Here's how the part is built. I have some questions about the finished solid (model axes, mm). Face numbers are marked on the shaded views. A direction names the side the tool comes from. Round coordinates to 2 decimals unless told otherwise and drop trailing zeros. Loops run counter-clockwise (first coordinate to the right, second up) from the corner with the lowest first, then second, coordinate; pieces in that order, holes last. Notation, with made-up numbers: (-2, 50.5) - (26, 50.5) arc R26 ccw to (26, 86.5) - close; hole circle Ø11 at (50, 57.5). An arc over 180 degrees is marked (long way). Return JSON: item names as keys, results as strings. Group by question number.
Autodesk Inventor part; units mm, degrees
ref_plane "YZ Plane" through (0, 0, 0) normal (1, 0, 0) x (0, 1, 0)
ref_plane "XZ Plane" through (0, 0, 0) normal (0, 1, 0) x (-1, 0, 0)
ref_plane "XY Plane" through (0, 0, 0) normal (0, 0, 1) x (1, 0, 0)
sketch "Sketch1" plane through (0, 0, 0) normal (0, 0, 1) x (1, 0, 0)
  line L0 (0, 0) -> (-61.1827, -8.0012) construction
  line L1 (61.2899, -8.1227) -> (0, 0) construction
  line L2 (86.7988, -11.5034) -> (67.2983, -8.919)
  line L3 (-67.1847, -8.7862) -> (-86.5468, -11.3183)
  line L4 (0, 0) -> (0, -62.0753) construction
  line L5 (61.2899, -8.1227) -> (0, -62.0753) construction
  line L6 (-61.1827, -8.0012) -> (0, -62.0753) construction
  arc A0 (-29.7125, -39.3071) -> (-39.2375, -29.7799) centre (-39.2375, -39.3049) ccw
  arc A1 (-60.1692, -13.6752) -> (-55.9036, -26.1177) centre (0, 0) ccw
  arc A2 (56.0545, -26.1271) -> (60.2727, -13.8035) centre (0.1394, -0.1047) ccw
  line L7 (-50.1505, -29.7799) -> (-39.2375, -29.7799)
  line L8 (-29.7125, -39.3071) -> (-29.7151, -50.2201)
  arc A3 (39.3667, -29.7672) -> (29.6251, -39.4816) centre (39.3395, -39.4816) ccw
  line L9 (29.6251, -39.4816) -> (29.6251, -50.3946)
  line L10 (39.3667, -29.7672) -> (50.2797, -29.7978)
  circle A4 centre (0.1394, -0.1047) radius 55.5625 construction
  line L11 (-39.2375, -39.3049) -> (0.1394, -0.1047) construction
  line L12 (0.1394, -0.1047) -> (39.3395, -39.4816) construction
  line L13 (39.3395, -39.4816) -> (0, -62.0753) construction
  line L14 (-39.2375, -39.3049) -> (0, -62.0753) construction
  circle A5 centre (-39.2375, -39.3049) radius 2.4384
  circle A6 centre (39.3395, -39.4816) radius 2.4384
  arc A7 (-91.9453, -18.8835) -> (-85.1324, -39.6138) centre (0.1394, -0.1047) ccw
  arc A8 (-76.9964, -53.7918) -> (-8.2199, -93.7122) centre (0.1394, -0.1047) ccw
  arc A9 (8.2102, -93.7375) -> (77.1094, -54.0293) centre (0.1394, -0.1047) ccw
  arc A10 (83.8051, -42.9099) -> (92.1837, -19.0805) centre (0.1394, -0.1047) ccw
  line L15 (-93.0629, -12.1704) -> (-83.6165, -42.7332) construction
  line L16 (-78.9151, -50.9242) -> (-4.7625, -93.9568) construction
  line L17 (4.7625, -93.9709) -> (79.0426, -51.1588) construction
  line L18 (83.8051, -42.9099) -> (93.316, -12.3671) construction
  line L19 (0, -62.0753) -> (0, -103.9027) construction
  line L20 (-4.7625, -90.5498) -> (-4.7625, -86.0193)
  line L21 (4.7625, -86.0193) -> (4.7625, -90.5743)
  arc A11 (4.7625, -86.0193) -> (-4.7625, -86.0193) centre (0, -86.0193) ccw
  line L22 (0.1394, -0.1047) -> (81.6013, -47.1368) construction
  line L23 (83.8051, -42.9099) -> (76.9144, -38.9315)
  line L24 (72.1519, -47.1804) -> (76.0966, -49.4579)
  arc A12 (76.9144, -38.9315) -> (72.1519, -47.1804) centre (74.5331, -43.0559) ccw
  line L25 (0.1394, -0.1047) -> (-92.6905, -53.7001) construction
  line L26 (-80.6641, -41.0286) -> (-76.7766, -38.7842)
  line L27 (-72.0545, -46.9632) -> (-75.978, -49.2284)
  arc A13 (-72.0545, -46.9632) -> (-76.7766, -38.7842) centre (-74.4155, -42.8737) ccw
  arc A14 (-86.5468, -11.3183) -> (-91.9453, -18.8835) centre (-85.7234, -17.6146) ccw
  arc A15 (-60.1692, -13.6752) -> (-67.1847, -8.7862) centre (-66.3613, -15.0825) ccw
  arc A16 (-55.9036, -26.1177) -> (-50.1505, -29.7799) centre (-50.1505, -23.4299) ccw
  arc A17 (-29.7151, -50.2201) -> (-25.945, -56.0239) centre (-23.3651, -50.2216) ccw
  arc A18 (25.7485, -56.2431) -> (29.6251, -50.3946) centre (23.2751, -50.3946) ccw
  arc A19 (50.2797, -29.7978) -> (56.0545, -26.1271) centre (50.2975, -23.4478) ccw
  arc A20 (67.2983, -8.919) -> (60.2727, -13.8035) centre (66.464, -15.2139) ccw
  arc A21 (92.1837, -19.0805) -> (86.7988, -11.5034) centre (85.9645, -17.7983) ccw
  arc A22 (-85.1324, -39.6138) -> (-80.6641, -41.0286) centre (-82.2516, -38.279) ccw
  arc A23 (-75.978, -49.2284) -> (-76.9964, -53.7918) centre (-74.3905, -51.9781) ccw
  arc A24 (-8.2199, -93.7122) -> (-4.7625, -90.5498) centre (-7.9375, -90.5498) ccw
  arc A25 (4.7625, -90.5743) -> (8.2102, -93.7375) centre (7.9375, -90.5743) ccw
  arc A26 (77.1094, -54.0293) -> (76.0966, -49.4579) centre (74.5091, -52.2075) ccw
  arc A27 (4.5025, -51.1894) -> (-4.48, -51.1668) centre (0, -55.667) ccw
  arc A28 (-25.945, -56.0239) -> (-15.3876, -59.8229) centre (0.1394, -0.1047) ccw
  arc A29 (15.3666, -59.9) -> (25.7485, -56.2431) centre (0.1394, -0.1047) ccw
  line L28 (-4.48, -51.1668) -> (-12.3487, -59.0002)
  line L29 (4.5025, -51.1894) -> (12.3318, -59.0621)
  arc A30 (-15.3876, -59.8229) -> (-12.3487, -59.0002) centre (-14.5887, -56.75) ccw
  arc A31 (12.3318, -59.0621) -> (15.3666, -59.9) centre (14.5831, -56.8232) ccw
  circle A32 centre (0, -55.667) radius 2.4384
  point P0 (-54.0417, -29.7799)
  point P1 (-29.716, -54.3478)
  point P2 (29.6251, -54.3566)
  point P3 (54.1888, -29.8087)
  point P4 (-13.611, -60.2568)
  point P5 (13.5878, -60.325)
  dimension "d2" = 165
  dimension "d5" = 9.525
  dimension "d7" = 111.125
  dimension "d8" = 4.8768
  dimension "d9" = 93.98
  dimension "d10" = 4.7625
  dimension "d11" = 60
  dimension "d12" = 7.9375
  dimension "d13" = 60
  dimension "d16" = 6.35
  dimension "d17" = 3.175
  dimension "d18" = 6.35
  dimension "d19" = 3.175
extrude "Extrusion3" add sketch "Sketch1" along normal blind 19.05
properties part number "IFI_Wheel_Weight_8in" material "Aluminum-6061"
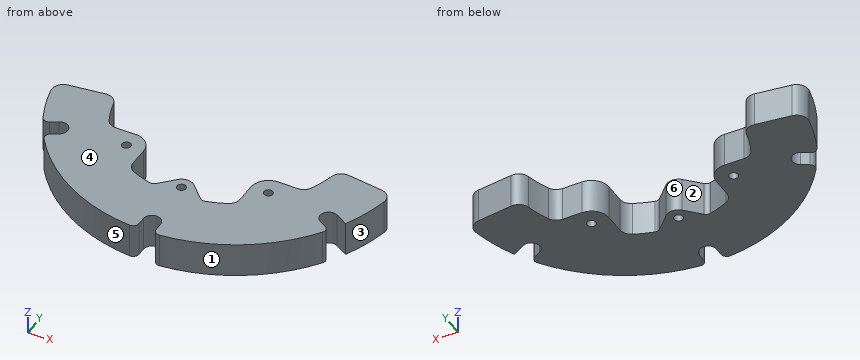
Q1. Imagine slicing it at D-D, the plane x = 52. List the corners of the cut face in (y, z) for me.
Q2. Please list where these lines run through material, in increasing order: line 1 (X direction, y = -42, z = 15); line 2 (Y direction, x = 0, z = 14.5); line 3 (X direction, y = -43, z = 9.75).
Q3. Will these pins go through, and if not, where does the flat tip stop? pin 1 Ø10 at (x, z) = (-51.5, 6) entering from -Y; pin 2 Ø1 at (y, z) = (-51, 6.5) entering from -X; pin 3 Ø10 at (x, z) = (-35, 4.5) entering from +Y.
Q4. If we mould it in two halves opening along X, with no side actions, what happens to the marked faces 3, 4, 5 and 6? For each: +X half, -X half, draft (parallel to the pull), parting line (faces both ways), or undercut.
Q5. Imagine slicing it at A-A, the plane x = 0. List the corners of the cut face in (y, z) for me, and give its area (3 significant figures).
Q6. For the marked faces 1 and 2, which set-ups out of +Z, -Z, +X, -X, +Y, -Y let a thin tool reach every point of the face, with its end or its side?
Q7. Imagine slicing it at C-C, the plane x = 81. List the corners of the cut face in (y, z) for me, and give its area (3 significant figures).
Q8. Imagine slicing it at B-B, the plane z = 15.5. Give the number of separate pieces and of enclosed holes in the cut face, and give its area (3 significant figures).
Output values:
{
 "1": {"outline": "(-78.48, 0) - (-29.57, 0) - (-29.57, 19.05) - (-78.48, 19.05) - close"},
 "2": {"line 1": "x = -69.77 to -29.71, 29.63 to 69.89, 82.23 to 84.26", "line 2": "y = -81.26 to -58.11, -53.23 to -49.32", "line 3": "x = -69.7 to -29.71, 29.63 to 69.77"},
 "3": {"pin 1": "stops at y = -81.7", "pin 2": "stops at x = -77.53", "pin 3": "stops at y = -29.78"},
 "4": {"face 3": "+X half", "face 4": "draft", "face 5": "-X half", "face 6": "undercut"},
 "5": {"outline": "(-81.26, 0) - (-58.11, 0) - (-58.11, 19.05) - (-81.26, 19.05) - close; (-53.23, 0) - (-49.32, 0) - (-49.32, 19.05) - (-53.23, 19.05) - close", "area": "516 mm^2"},
 "6": {"face 1": "+Z, -Z, +X, -Y", "face 2": "+Z, -Z, +Y"},
 "7": {"outline": "(-41.29, 0) - (-10.73, 0) - (-10.73, 19.05) - (-41.29, 19.05) - close", "area": "582 mm^2"},
 "8": {"separate pieces": "1", "enclosed holes": "3", "area": "7,690 mm^2"}
}
